from build123d import *

# Parameters (mm, degrees)
F0_W          = 10
F0_H          = 2
F1_DEPTH      = 2
F2_W          = 0.75
F2_H          = 0.75
F2_W_2        = 0.787472
F2_H_2        = 0.823894
F2_W_3        = 0.66187
F2_W_4        = 0.875056
F3_DEPTH      = 8.5
F3_DEPTH_BACK = 5
F4_SIZE       = 0.1
F5_SIZE       = 0.1
F6_SIZE       = 0.1
F7_SIZE       = 0.1
F8_SIZE       = 0.2


with BuildPart() as f1:
    # F0 (on Top) → F1 (new body)
    with BuildSketch(Plane.XY):
        Rectangle(F0_W, F0_H)
    extrude(amount=F1_DEPTH)

    # F2 (on face) → F3 (join, two sides)
    with BuildSketch(Plane.XY.offset(2)) as f3_sk:
        with Locations((-3.895019, -0.036947)):
            Rectangle(F2_W, F2_H)
        with Locations((-1.373755, 0)):
            Rectangle(F2_W_2, F2_H_2)
        with Locations((1.229046, 0)):
            Rectangle(F2_W_3, F2_H_2)
        with Locations((3.662453, 0)):
            Rectangle(F2_W_4, F2_H_2)
    extrude(amount=F3_DEPTH)
    extrude(f3_sk.sketch, amount=-F3_DEPTH_BACK)

    # F4
    f4_edges = [f1.edges().sort_by_distance(p)[0] for p in [
        (-3.895019, -0.411947, 10.5),
        (-3.520019, -0.036947, 10.5),
        (-3.895019, 0.338053, 10.5),
        (-4.270019, -0.036947, 10.5),
    ]]
    chamfer(f4_edges, length=F4_SIZE)

    # F5
    f5_edges = [f1.edges().sort_by_distance(p)[0] for p in [
        (-1.373755, -0.411947, 10.5),
        (-0.980019, 0, 10.5),
        (-1.373755, 0.411947, 10.5),
        (-1.767491, 0, 10.5),
    ]]
    chamfer(f5_edges, length=F5_SIZE)

    # F6
    f6_edges = [f1.edges().sort_by_distance(p)[0] for p in [
        (0.898111, 0, 10.5),
        (1.229046, -0.411947, 10.5),
        (1.559981, 0, 10.5),
        (1.229046, 0.411947, 10.5),
    ]]
    chamfer(f6_edges, length=F6_SIZE)

    # F7
    f7_edges = [f1.edges().sort_by_distance(p)[0] for p in [
        (3.224925, 0, 10.5),
        (3.662453, -0.411947, 10.5),
        (4.099981, 0, 10.5),
        (3.662453, 0.411947, 10.5),
    ]]
    chamfer(f7_edges, length=F7_SIZE)

    # F8
    f8_edges = [f1.edges().sort_by_distance(p)[0] for p in [
        (3.224925, 0, -3),
        (3.662453, -0.411947, -3),
        (4.099981, 0, -3),
        (3.662453, 0.411947, -3),
        (0.898111, 0, -3),
        (1.229046, -0.411947, -3),
        (1.559981, 0, -3),
        (1.229046, 0.411947, -3),
        (-1.373755, 0.411947, -3),
        (-1.767491, 0, -3),
        (-1.373755, -0.411947, -3),
        (-0.980019, 0, -3),
        (-3.520019, -0.036947, -3),
        (-3.895019, 0.338053, -3),
        (-4.270019, -0.036947, -3),
        (-3.895019, -0.411947, -3),
    ]]
    chamfer(f8_edges, length=F8_SIZE)


solid = f1.part
The listing builds one solid part. Answer for the finished solid, in the listing's coordinates (mm). A direction names the side the tool comes from. Give positions to 0.01 mm unless a question says otherwise; leave off trailing zeros. Loops run counter-clockwise (first coordinate to the right, second up) from the corner with the lowest first, then second, coordinate; pieces in that order, holes last. Notation, with made-up numbers: (17.25, -27.75) - (28.25, -27.75) arc R13 cw to (28.25, -22.75) - close; hole circle Ø10 at (32, -27.75). An arc over 180 degrees is marked (long way). Write each question's results on one line, items separated by ' | '.
1. Find section C-C, the plane x = 0.5. Write down the section's boundary in (y, z).
Resolved:
outline: (-1, 0) - (1, 0) - (1, 2) - (-1, 2) - close
2. Consider probe 1 along X at (y, z) = (0.1, 6); probe 2 along Y at (x, z) = (4, 9.5); probe 3 along Z at (x, y) = (-1.75, 0.8). Determine where each line is inside the solid, lowest interval first. Write a range as from..to.
Resolved:
probe 1: x = -4.27..-3.52, -1.77..-0.98, 0.9..1.56, 3.22..4.1 | probe 2: y = -0.41..0.41 | probe 3: z = 0..2
3. Flat-ended cylindrical pins translate along their axes: P1, Ø0.6, axis at x = -1.5, z = -1, coming from the -Y side; P2, Ø0.8, axis at x = -4, z = 5, coming from the +Y side; P3, Ø0.9, axis at x = -1.5, z = 8, coming from the +Y side. Find the tip coordinate at first contact, or state that the pin passes through.
Resolved:
P1: stops at y = -0.41 | P2: stops at y = 0.34 | P3: stops at y = 0.41
4. Find section A-A, the plane z = 9.75. Write down the section's boundary in (x, y), then the cut area to 3 significant figures.
Resolved:
outline: (-4.27, -0.41) - (-3.52, -0.41) - (-3.52, 0.34) - (-4.27, 0.34) - close; (-1.77, -0.41) - (-0.98, -0.41) - (-0.98, 0.41) - (-1.77, 0.41) - close; (0.9, -0.41) - (1.56, -0.41) - (1.56, 0.41) - (0.9, 0.41) - close; (3.22, -0.41) - (4.1, -0.41) - (4.1, 0.41) - (3.22, 0.41) - close | area: 2.48 mm^2
5. Which of the six approach directions +Z, -Z, +X, -X, +Y, -Y give full straight-line access (tool end or side, diameter ignored) to faces 1 (the face through (1.56, 0, 6)), 2 (the face through (4.1, 0, 6)), 3 (the face through (3.225, 0, -1))?
Resolved:
face 1: +Z, +Y, -Y | face 2: +Z, +X, +Y, -Y | face 3: -Z, +Y, -Y
6. Find section B-B, the plane y = -0.65. Write down the section's boundary in (x, z).
Resolved:
outline: (-5, 0) - (5, 0) - (5, 2) - (-5, 2) - close
7. For a pull along X with two mould halves and no side action, classify faces 4 (the face through (0.898, 0, -1)), 5 (the face through (3.7, 0.412, 6.1)), 6 (the face through (5, 0, 1)) as +X half, -X half, draft (parallel to the pull), parting line (faces both ways), or undercut.
Resolved:
face 4: undercut | face 5: draft | face 6: +X half
